```python
from build123d import *


# Read off the part's stored shape, not the designer's step: 抽壳1
with BuildPart() as part:
    # 草图1 → 旋转1 (revolve)
    with BuildSketch(Plane.XY, mode=Mode.PRIVATE) as revolve_1_sk:
        with BuildLine():
            Line((0, 129.302861252), (0, -165.697138748))
            Line((0, -165.697138748), (25.5, -165.697138748))
            ThreePointArc((25.5, -165.697138748), (29.035533906, -164.232672654), (30.5, -160.697138748))
            Line((30.5, -160.697138748), (30.5, 74.302861252))
            ThreePointArc((30.5, 74.302861252), (27.22407628, 92.146010239), (17.823593149, 107.661826649))
            ThreePointArc((17.823593149, 107.661826649), (15.952164194, 110.750683646), (15.3, 114.302861252))
            Line((15.3, 114.302861252), (15.3, 127.302861252))
            ThreePointArc((15.3, 127.302861252), (14.714213562, 128.717074815), (13.3, 129.302861252))
            Line((13.3, 129.302861252), (0, 129.302861252))
        make_face()
    revolve(revolve_1_sk.sketch.rotate(Axis((0, 129.302861252, 0), (0, -1, 0)), 180), axis=Axis((0, 129.302861252, 0), (0, -1, 0)))

    # 抽壳1 outline → 抽壳1 (revolve, cut)
    with BuildSketch(Plane.XY):
        with BuildLine():
            Line((0, -159.397138748), (24.2, -159.397138748))
            Line((24.2, -159.397138748), (24.2, 74.302861252))
            ThreePointArc((24.2, 74.302861252), (21.334939722, 89.908138347), (13.113456833, 103.477974849))
            ThreePointArc((13.113456833, 103.477974849), (10.063027636, 108.512811754), (9, 114.302861252))
            Line((9, 114.302861252), (9, 129.302861252))
            Line((9, 129.302861252), (0, 129.302861252))
            Line((0, 129.302861252), (0, -159.397138748))
        make_face()
    revolve(axis=Axis((0, 0, 0), (0, 1, 0)), mode=Mode.SUBTRACT)


solid = part.part
```
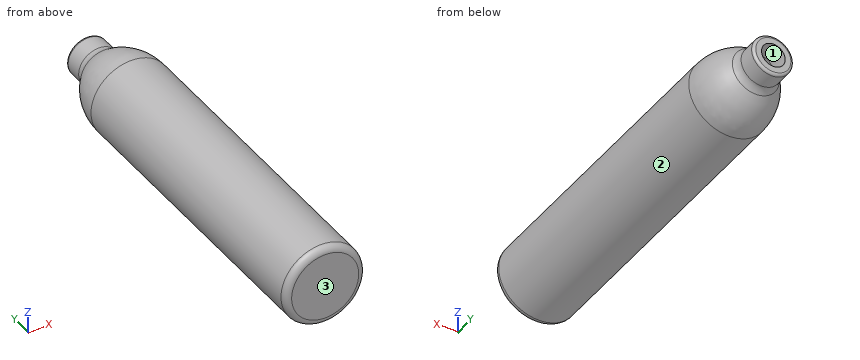
The listing builds one solid part. Answer for the finished solid, in the listing's coordinates (mm). Face numbers are marked on the shaded views. Give positions to 0.01 mm unless a question says otherwise; leave off trailing zeros. Loops run counter-clockwise (first coordinate to the right, second up) from the corner with the lowest first, then second, coordinate; pieces in that order, holes last. Notation, with made-up numbers: (65.5, -12.5) - (83.5, -12.5) arc R11 cw to (83.5, -1.5) - close; hole circle Ø6 at (20, -19.75). An arc over 180 degrees is marked (long way). Return JSON: item names as keys, results as strings. Group by question number.
1. Find section A-A (y = -12.5). Write down the section's boundary in (x, z).
2. Straight lines are drawn through the part: line 1 (Z direction, x = 0, y = 124); line 2 (Z direction, x = 0, y = -97); line 3 (Y direction, x = -16.5, z = -11.5). For each, find the intervals that lie inside material, in ascending order. Write a range as [from, to].
3. Given pin 1 Ø10 at (x, z) = (23.5, -16.5) entering from +Y; pin 2 Ø10 at (x, y) = (21, 65.5) entering from +Z; pin 3 Ø5 at (x, y) = (16, -6.5) entering from +Z, each flat-ended and moving along its own axis, determine where each tip first touches the part or whether it passes through.
4. Determine the mould class of the marked faces 1, 2 and 3 for opening direction X: pulls with the +X half, pulls with the -X half, needs draft (parallel to the pull), parting line crosses it, or undercut.
Verdict:
{
 "1": {"outline": "circle Ø61 at (0, 0); hole circle Ø48.4 at (0, 0)"},
 "2": {"line 1": "z = [-15.3, -9], [9, 15.3]", "line 2": "z = [-30.5, -24.2], [24.2, 30.5]", "line 3": "y = [-165.7, -159.4], [92.81, 104.89]"},
 "3": {"pin 1": "stops at y = 99.52", "pin 2": "stops at z = 25.97", "pin 3": "stops at z = 27.35"},
 "4": {"face 1": "undercut", "face 2": "parting line crosses it", "face 3": "needs draft"}
}
